Design review of the part built by this model. Coordinates are the model's own, in mm. Coordinates: 2 decimals unless noted, no trailing zeros. Order: outer loops, then holes, each group sorted by start corner. A loop starts at its lowest first (then second) coordinate and runs counter-clockwise, first axis right, second up.
from build123d import *

# Parameters (mm, degrees)
SKETCH1_W           = 50.8
SKETCH1_H           = 50.8
BOSS_EXTRUDE1_DEPTH = 6.35
SKETCH2_R           = 9.906
CUT_EXTRUDE1_DEPTH  = 7.35
SKETCH3_R           = 1.27
CUT_EXTRUDE2_DEPTH  = 7.35
CIRPATTERN1_COUNT   = 3
FILLET1_R           = 6.35


with BuildPart() as part:
    # Sketch1 → Boss-Extrude1 (new body)
    with BuildSketch(Plane(origin=(0, 0, 0), x_dir=(1, 0, 0), z_dir=(0, 1, 0))):
        Rectangle(SKETCH1_W, SKETCH1_H)
    extrude(amount=BOSS_EXTRUDE1_DEPTH)

    # Sketch2 → Cut-Extrude1 (cut, through all)
    with BuildSketch(Plane(origin=(0, 6.35, 0), x_dir=(1, 0, 0), z_dir=(0, 1, 0))):
        Circle(SKETCH2_R)
    extrude(amount=-CUT_EXTRUDE1_DEPTH, mode=Mode.SUBTRACT)

    # Sketch3 → Cut-Extrude2 (cut, through all)
    with BuildSketch(Plane(origin=(0, 6.35, 0), x_dir=(1, 0, 0), z_dir=(0, 1, 0))):
        with Locations((12.7, 0)):
            Circle(SKETCH3_R)
    cut_extrude2 = extrude(amount=-CUT_EXTRUDE2_DEPTH, mode=Mode.SUBTRACT)

    # CirPattern1: Cut-Extrude2 ×3 about axis
    cirpattern1_axis = Axis((0, 0, 0), (0, 1, 0))
    for i in range(1, CIRPATTERN1_COUNT):
        add(cut_extrude2.rotate(cirpattern1_axis, i * 360 / CIRPATTERN1_COUNT), mode=Mode.SUBTRACT)

    # Fillet1
    fillet1_edges = [part.edges().sort_by_distance(p)[0] for p in [
        (25.4, 3.175, 25.4),
        (-25.4, 3.175, 25.4),
        (-25.4, 3.175, -25.4),
        (25.4, 3.175, -25.4),
    ]]
    fillet(fillet1_edges, radius=FILLET1_R)


solid = part.part
1. Mouldability with a two-part tool opening along X and no side actions: class faces 1 (the flat face through (0, 3, -25.4)), 2 (the cylindrical face through (23.49, 3.22, 23.59)), 3 (the cylindrical face through (-23.59, 3.22, 23.49)), 4 (the cylindrical face through (-1.29, 3.22, -9.82)) as pulls with the +X half, pulls with the -X half, needs draft (parallel to the pull), parting line crosses it, or undercut.
2. Insertion check: pin 1 (1.5 mm diameter, centred on x = -20, y = 5.5, fed in from +Z); pin 2 (3 mm diameter, centred on x = -6.35, z = -11, fed in from -Y); pin 3 (18 mm diameter, centred on x = 0, z = 0, fed in from +Y). Each pin has a flat end and moves straight along its axis. Give the tip position at first contact, or say it passes through.
3. To check wall thickness, follow line 1 (X direction, y = 4.25, z = 0); line 2 (X direction, y = 1.5, z = -11); line 3 (Z direction, x = -6.35, y = 4.25). State the ranges of each line that lie inside material, in increasing order.
4. Add section B-B (x = 12.7). Give the boundary of the cut face in (y, z).
5. Add section D-D (x = -6.35). Give the boundary of the cut face in (y, z).
6. Add section A-A (z = 0). Give the boundary of the cut face in (x, y), and give its area (3 significant figures).
7. Add section C-C (z = 7.5). Give the boundary of the cut face in (x, y), and give its area (3 significant figures).
Solution:
1. face 1: needs draft
1. face 2: pulls with the +X half
1. face 3: pulls with the -X half
1. face 4: undercut
2. pin 1: stops at z = 25.4
2. pin 2: stops at y = 0
2. pin 3: passes through
3. line 1: x = -25.4 to -9.91, 9.91 to 11.43, 13.97 to 25.4
3. line 2: x = -25.4 to -7.62, -5.08 to 25.4
3. line 3: z = -25.4 to -12.27, -9.73 to -7.6, 7.6 to 9.73, 12.27 to 25.4
4. outline: (0, -25.4) - (6.35, -25.4) - (6.35, -1.27) - (0, -1.27) - close; (0, 1.27) - (6.35, 1.27) - (6.35, 25.4) - (0, 25.4) - close
5. outline: (0, -25.4) - (6.35, -25.4) - (6.35, -12.27) - (0, -12.27) - close; (0, -9.73) - (6.35, -9.73) - (6.35, -7.6) - (0, -7.6) - close; (0, 7.6) - (6.35, 7.6) - (6.35, 9.73) - (0, 9.73) - close; (0, 12.27) - (6.35, 12.27) - (6.35, 25.4) - (0, 25.4) - close
6. outline: (-25.4, 0) - (-9.91, 0) - (-9.91, 6.35) - (-25.4, 6.35) - close; (9.91, 0) - (11.43, 0) - (11.43, 6.35) - (9.91, 6.35) - close; (13.97, 0) - (25.4, 0) - (25.4, 6.35) - (13.97, 6.35) - close
6. area: 181 mm2
7. outline: (-25.4, 0) - (-6.47, 0) - (-6.47, 6.35) - (-25.4, 6.35) - close; (6.47, 0) - (25.4, 0) - (25.4, 6.35) - (6.47, 6.35) - close
7. area: 240 mm2
